Job drawing, mm, ordinate dimensions from the low corner. One solid piece. A direction names the side the tool comes from. Give positions to 0.01 mm unless a question says otherwise; leave off trailing zeros. Loops run counter-clockwise (first coordinate to the right, second up) from the corner with the lowest first, then second, coordinate; pieces in that order, holes last.
Item 1: Drop flat-ended pins along their axis: P1, Ø2.5, axis at y = 42, z = 42.5, coming from the -X side; P2, Ø2.5, axis at y = 40, z = 42.5, coming from the +X side; P3, Ø5.5, axis at x = 22.5, z = 13, coming from the +Y side; P4, Ø2.5, axis at x = 6, z = 31, coming from the -Y side. Give the stop position or say it passes through.
Item 2: Mould opens along Z. For the marked faces 1, 2, 3 and 4 say: released by +Z, released by -Z, zero draft, split by the parting line, or undercut.
Item 3: Saw through at C-C on y = 43. Give the cut face in (x, z), plus the area to 3 significant figures.
Item 4: Saw through at A-A on y = 23. Give the cut face in (x, z).
Item 5: Probe probe 1 along X at (y, z) = (2.7, 31); probe 2 along Z at (x, y) = (20, 36.5); probe 3 along Z at (x, y) = (26.5, 28). List the from-to ranges inside material, lowest first.
Item 6: Saw through at B-B on z = 31. Give the cut face in (x, y), plus the area to 3 significant figures.
Item 7: Which spindle directions (+Z, -Z, +X, -X, +Y, -Y) get a long thin tool onto all of the face, cutting with end or side? Do the marked faces 5 and 6. Say none if no direction does.
Item 8: Saw through at D-D on x = 2. Give the cut face in (y, z).
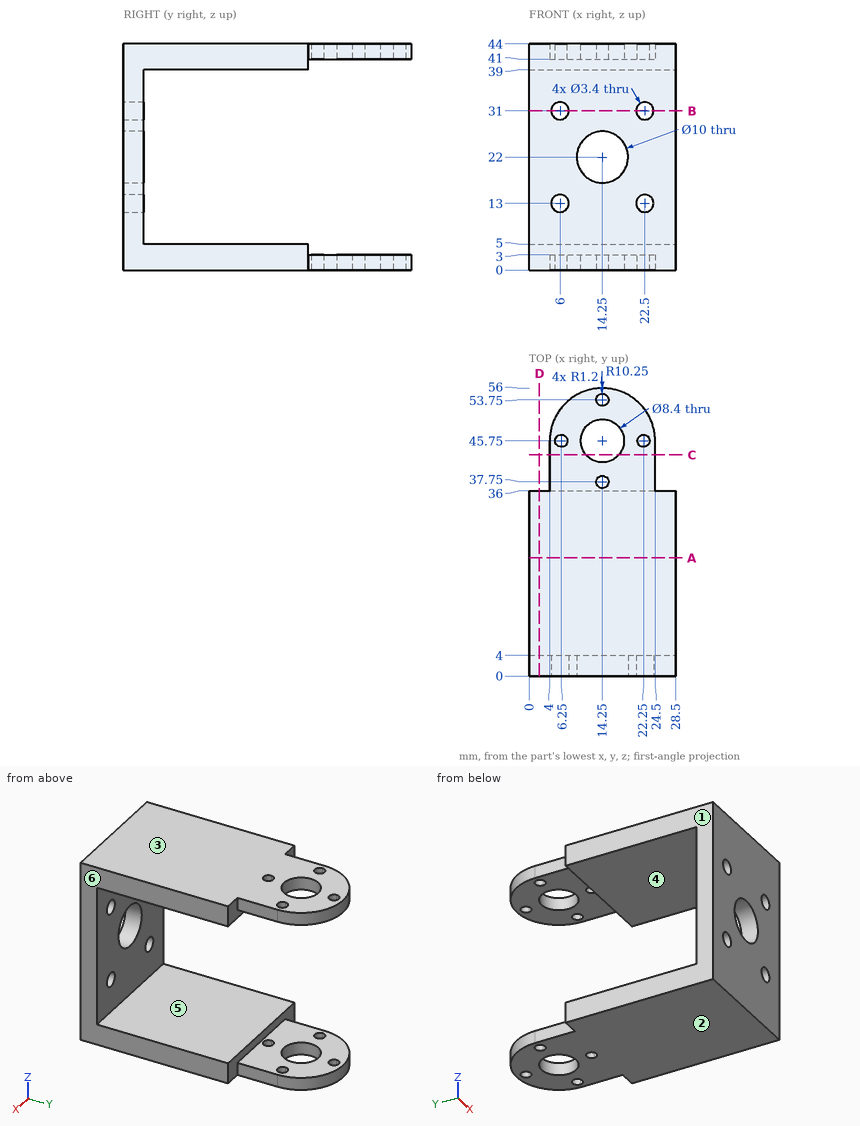
Results below:
1. P1: stops at x = 4
1. P2: stops at x = 24.5
1. P3: stops at y = 4
1. P4: passes through
2. face 1: zero draft
2. face 2: released by -Z
2. face 3: released by +Z
2. face 4: undercut
3. outline: (4, 0) - (11.08, 0) - (11.08, 3) - (4, 3) - close; (4, 41) - (11.08, 41) - (11.08, 44) - (4, 44) - close; (17.42, 0) - (24.5, 0) - (24.5, 3) - (17.42, 3) - close; (17.42, 41) - (24.5, 41) - (24.5, 44) - (17.42, 44) - close
3. area: 84.9 mm2
4. outline: (0, 0) - (28.5, 0) - (28.5, 5) - (0, 5) - close; (0, 39) - (28.5, 39) - (28.5, 44) - (0, 44) - close
5. probe 1: x = 0 to 4.3, 7.7 to 20.8, 24.2 to 28.5
5. probe 2: z = 0 to 3, 41 to 44
5. probe 3: z = 0 to 5, 39 to 44
6. outline: (0, 0) - (4.3, 0) - (4.3, 4) - (0, 4) - close; (7.7, 0) - (20.8, 0) - (20.8, 4) - (7.7, 4) - close; (24.2, 0) - (28.5, 0) - (28.5, 4) - (24.2, 4) - close
6. area: 86.8 mm2
7. face 5: +X, -X, +Y
7. face 6: +Z, -Z, +X, +Y, -Y
8. outline: (0, 0) - (36, 0) - (36, 5) - (4, 5) - (4, 39) - (36, 39) - (36, 44) - (0, 44) - close
